Autodesk Inventor part; units mm, degrees
ref_plane "YZ Plane" through (0, 0, 0) normal (1, 0, 0) x (0, 1, 0)
ref_plane "XZ Plane" through (0, 0, 0) normal (0, 1, 0) x (-1, 0, 0)
ref_plane "XY Plane" through (0, 0, 0) normal (0, 0, 1) x (1, 0, 0)
sketch "Sketch1" plane through (0, 0, 0) normal (0, 1, 0) x (-1, 0, 0)
  line L0 (0, 0) -> (50, 0)
  line L1 (50, 0) -> (50, -300)
  line L2 (50, -300) -> (0, -300)
  line L3 (0, -300) -> (0, 0)
  dimension "d0" = 50
  dimension "d1" = 300
extrude "Extrusion1" add sketch "Sketch1" along normal blind 80
sketch "Sketch2" plane through (0, 80, 0) normal (0, 1, 0) x (1, 0, 0)
  line L0 (0, 0) -> (-50, 0)
  line L1 (-50, 0) -> (-50, 150)
  line L2 (-50, 150) -> (0, 150)
  line L3 (0, 150) -> (0, 0)
  dimension "d4" = 50
  dimension "d5" = 150
extrude "Extrusion2" cut sketch "Sketch2" against normal blind 100
sketch "Sketch3" plane through (0, 80, 0) normal (0, 1, 0) x (1, 0, 0)
  line L0 (-44.983, 155.2795) -> (-4.983, 155.2795)
  line L1 (-4.983, 155.2795) -> (-4.983, 295.2795)
  line L2 (-4.983, 295.2795) -> (-44.983, 295.2795)
  line L3 (-44.983, 295.2795) -> (-44.983, 155.2795)
  point P0 (0, 0)
  dimension "d8" = 40
  dimension "d9" = 140
extrude "Extrusion3" cut sketch "Sketch3" against normal blind 70
properties part number "storebox2"
Here's how the part is built. I have some questions about the finished solid (model axes, mm). A direction names the side the tool comes from. Give positions to 0.01 mm unless a question says otherwise; leave off trailing zeros. Loops run counter-clockwise (first coordinate to the right, second up) from the corner with the lowest first, then second, coordinate; pieces in that order, holes last. Notation, with made-up numbers: (-7, 69) -> (20, 69) arc R15 cw to (20, 76) -> close; hole circle Ø8 at (-35, 80). An arc over 180 degrees is marked (long way). Use one line per item in the form item = value. Start each with the question number.
1) Imagine slicing it at B-B (z = -190). Please give me the cut outline in (x, y), then the cut area to 3 significant figures.
2) Imagine slicing it at A-A (y = 42). Please give me the cut outline in (x, z), then the cut area to 3 significant figures.
3) Thinking about a two-plate mould opening in Z: for faces 3 (the face through (-25, 39, -300)), 4 (the face through (-50, 39, -224)), 5 (the face through (-25, 45, -295.28)), which applies, +Z half, -Z half, draft (parallel to the pull), parting line (faces both ways), or undercut?
4) For P1, Ø1, axis at x = -30, z = -178, coming from the +Y side; P2, Ø8, axis at y = 29.5, z = -191, coming from the +X side, each with a flat end and sliding along its axis, tell me the tip position at first contact or that it passes through.
5) Which directions (+Z, -Z, +X, -X, +Y, -Y) give clear straight access to the entire face, cutting with the end or side of a thin tool? Please do faces 1 (the face through (-25, 10, -226)), 2 (the face through (-4.5, 80, -219.1)).
6) Please list where these lines run through material, in increasing order: line 1 along Z through (x, y) = (-21, 44); line 2 along X through (y, z) = (12.5, -277); line 3 along Y through (x, z) = (-34.5, -277.5).
7) Imagine slicing it at C-C (x = -25.5). Please give me the cut outline in (y, z), then the cut area to 3 significant figures.
Check values:
q1.outline = (-50, 0) -> (0, 0) -> (0, 80) -> (-4.98, 80) -> (-4.98, 10) -> (-44.98, 10) -> (-44.98, 80) -> (-50, 80) -> close
q1.area = 1,200 mm^2
q2.outline = (-50, -300) -> (0, -300) -> (0, -150) -> (-50, -150) -> close; hole (-44.98, -295.28) -> (-4.98, -295.28) -> (-4.98, -155.28) -> (-44.98, -155.28) -> close
q2.area = 1,900 mm^2
q3.face_3 = -Z half
q3.face_4 = draft
q3.face_5 = undercut
q4.P1 = 10
q4.P2 = 0
q5.face_1 = +Y
q5.face_2 = +Z, -Z, +X, -X, +Y
q6.line_1 = -300 to -295.28, -155.28 to -150
q6.line_2 = -50 to -44.98, -4.98 to 0
q6.line_3 = 0 to 10
q7.outline = (0, -300) -> (80, -300) -> (80, -295.28) -> (10, -295.28) -> (10, -155.28) -> (80, -155.28) -> (80, -150) -> (0, -150) -> close
q7.area = 2,200 mm^2
